Job drawing, mm, ordinate dimensions from the low corner. One solid piece. A direction names the side the tool comes from. Give positions to 0.01 mm unless a question says otherwise; leave off trailing zeros. Write each loop counter-clockwise with the first axis right and the second up, starting at its lowest first coordinate (ties: lowest second). Pieces come first, ordered by that corner, then holes. Notation, with made-up numbers: M 57,38 L 94,38 A30 ccw 94,74 Z; hole C 55.25,-18 d10. An arc over 180 degrees is marked long. Answer as CSV lines item,"result". Start each with the question number.
Item 1: Pin check, flat tips, straight feed: pin 1 (5 mm diameter, centred on x = 9, y = 20, fed in from +Z); pin 2 (2 mm diameter, centred on x = 6.5, z = 3, fed in from -Y); pin 3 (1.5 mm diameter, centred on x = 8.5, y = 21.5, fed in from -Z); pin 4 (4 mm diameter, centred on x = 4, z = 2, fed in from +Y). Stop position of each tip, or through.
Item 2: Two-plate mould, pull along Y, no slides. Class the marked faces 1, 2 and 3: +Y half, -Y half, draft (parallel to the pull), parting line (faces both ways), or undercut.
Item 3: Band-saw the part on A-A, the plane z = 6.5. List the corners of the cut face in (x, y).
Item 4: Band-saw the part on D-D, the plane z = 1.75. List the corners of the cut face in (x, y), then the cut area to 3 significant figures.
Item 5: 3-axis set-ups, long thin cutter, end or side, ignore diameter. For the marked faces 4, 5, 6, 7 and 8: which of +Z, -Z, +X, -X, +Y, -Y reach the whole face in a straight line?
Item 6: Band-saw the part on C-C, the plane x = 12.5. List the corners of the cut face in (y, z), then the cut area to 3 significant figures.
Item 7: Band-saw the part on B-B, the plane x = 16. List the corners of the cut face in (y, z), then the cut area to 3 significant figures.
Item 8: Wall check: L1, parallel to Y at x = 12, z = 6.75; L2, parallel to Y at x = 7.7, z = 0.5; L3, parallel to Z at x = 6.25, y = 28. Give the ranges that are in metal, low to high. Write a range as from..to.
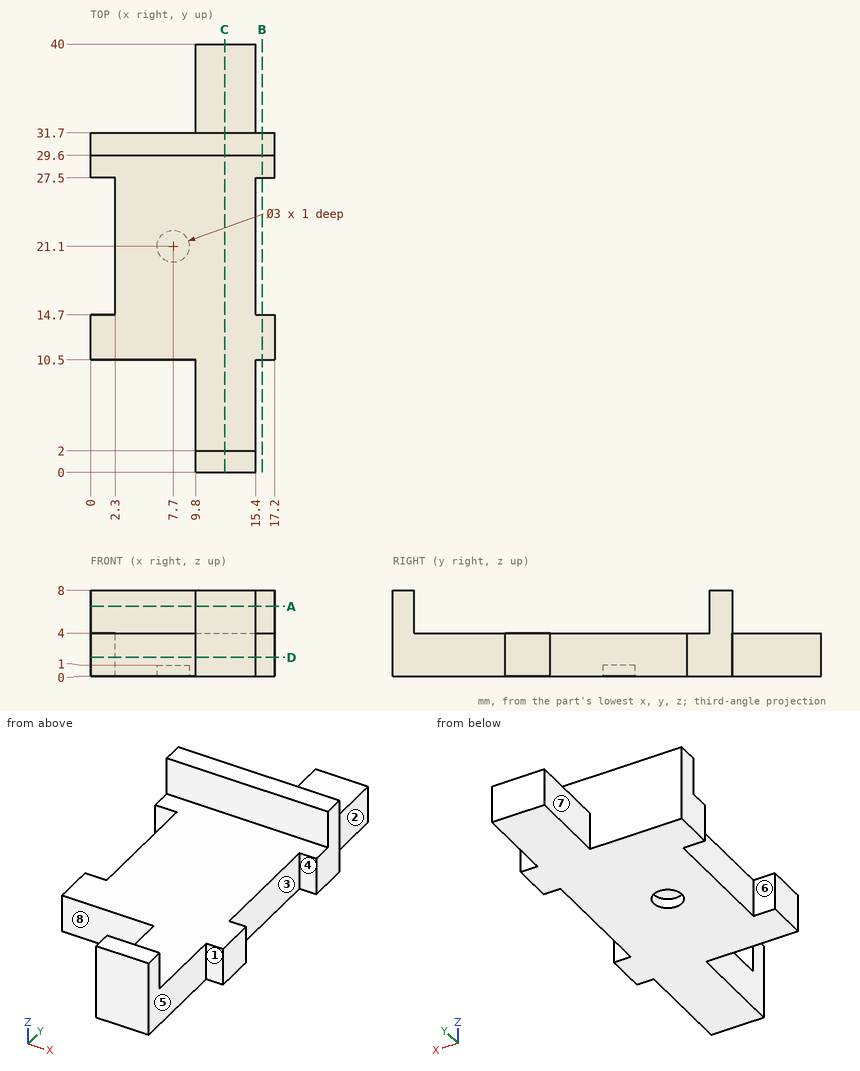
Output:
1,pin 1,"z = 4"
1,pin 2,"y = 10.5"
1,pin 3,"z = 0"
1,pin 4,"y = 31.7"
2,face 1,"-Y half"
2,face 2,"draft"
2,face 3,"undercut"
3,outline,"M 0,29.6 L 17.2,29.6 L 17.2,31.7 L 0,31.7 Z; M 9.8,0 L 15.4,0 L 15.4,2 L 9.8,2 Z"
4,outline,"M 0,10.5 L 9.8,10.5 L 9.8,0 L 15.4,0 L 15.4,10.5 L 17.2,10.5 L 17.2,14.7 L 15.4,14.7 L 15.4,27.5 L 17.2,27.5 L 17.2,31.7 L 15.4,31.7 L 15.4,40 L 9.8,40 L 9.8,31.7 L 0,31.7 L 0,27.5 L 2.3,27.5 L 2.3,14.7 L 0,14.7 Z"
4,area,"417 mm²"
5,face 4,"+Z, -Z, +X"
5,face 5,"+Z, -Z, +X, -Y"
5,face 6,"+Z, -Z, -X"
5,face 7,"+Z, -Z, -X, +Y"
5,face 8,"+Z, -Z, -X, -Y"
6,outline,"M 0,0 L 40,0 L 40,4 L 31.7,4 L 31.7,8 L 29.6,8 L 29.6,4 L 2,4 L 2,8 L 0,8 Z"
6,area,"176 mm²"
7,outline,"M 10.5,0 L 14.7,0 L 14.7,4 L 10.5,4 Z; M 27.5,0 L 31.7,0 L 31.7,8 L 29.6,8 L 29.6,4 L 27.5,4 Z"
7,area,"42.0 mm²"
8,L1,"0..2, 29.6..31.7"
8,L2,"10.5..19.6, 22.6..31.7"
8,L3,"0..4"
